Read the model definition and answer for the solid it produces. Units are mm, in the model's axes. A direction names the side the tool comes from. Coordinates: 2 decimals unless noted, no trailing zeros. Order: outer loops, then holes, each group sorted by start corner. A loop starts at its lowest first (then second) coordinate and runs counter-clockwise, first axis right, second up. Notation, with made-up numbers: M 68,1.25 L 97,1.25 A15 cw 97,10.25 Z; hole C 85,44.5 d10. An arc over 180 degrees is marked long. Write each question's results on one line, items separated by ' | '.
```python
from build123d import *

# Parameters (mm, degrees)
SKETCH_1_W             = 280
SKETCH_1_H             = 290
EXTRUDE_1_DEPTH        = 3
SKETCH_2_W             = 42
SKETCH_2_H             = 42
CUT_EXTRUDE_1_DEPTH    = 3
SKETCH_3_W             = 122
SKETCH_3_H             = 10
EXTRUDE_4_DEPTH        = 20
SKETCH_5_W             = 5
SKETCH_5_H             = 40
EXTRUDE_7_DEPTH        = 20
EXTRUDE_8_DEPTH        = 10
PATTERN_LINEAR_1_COUNT = 4
PATTERN_LINEAR_1_PITCH = 37.3
SKETCH_7_W             = 100
SKETCH_7_H             = 20
CUT_EXTRUDE_3_DEPTH    = 3
PATTERN_LINEAR_2_COUNT = 9
PATTERN_LINEAR_2_PITCH = 30
SKETCH_8_W             = 19.372377966
SKETCH_8_H             = 34.870206367
SKETCH_8_W_2           = 28.060398732
SKETCH_8_W_3           = 26.290591332
SKETCH_8_W_4           = 22.27663197
SKETCH_8_H_2           = 37.129793633
CUT_EXTRUDE_4_DEPTH    = 3


with BuildPart() as part:
    # 草图1 → 凸台-拉伸1 (new body)
    with BuildSketch(Plane(origin=(0, 0, 0), x_dir=(0, 0, -1), z_dir=(1, 0, 0))):
        with Locations((101.929406601, -104.613945148)):
            Rectangle(SKETCH_1_W, SKETCH_1_H)
    extrude(amount=EXTRUDE_1_DEPTH)

    # 草图2 → 切除-拉伸1 (cut)
    with BuildSketch(Plane.ZY):
        with Locations((-154.017718623, -48.907355815)):
            Rectangle(SKETCH_2_W, SKETCH_2_H)
    extrude(amount=-CUT_EXTRUDE_1_DEPTH, mode=Mode.SUBTRACT)

    # 草图3 → 凸台-拉伸4 (add)
    with BuildSketch(Plane.ZY):
        with Locations((-155.503619283, -115.067977161)):
            Rectangle(SKETCH_3_W, SKETCH_3_H)
    extrude(amount=EXTRUDE_4_DEPTH)

    # 草图5 → 凸台-拉伸7 (add)
    with BuildSketch(Plane.ZY):
        with Locations((-219.003619283, -10.067977161)):
            Rectangle(SKETCH_5_W, SKETCH_5_H)
        with Locations((-92.003619283, -10.067977161)):
            Rectangle(SKETCH_5_W, SKETCH_5_H)
    extrude(amount=EXTRUDE_7_DEPTH)

    # 草图6 → 凸台-拉伸8 (add)
    with BuildSketch(Plane.XY.offset(-94.503619283)):
        Polygon((-20, -120.067977161), (0, -120.067977161), (0, -140.067977161), align=None)
    extrude_8 = extrude(amount=-EXTRUDE_8_DEPTH)

    # 阵列(线性)1: 凸台-拉伸8 ×4
    with Locations(*[(0, 0, -i * PATTERN_LINEAR_1_PITCH) for i in range(1, PATTERN_LINEAR_1_COUNT)]):
        add(extrude_8)

    # 草图7 → 切除-拉伸3 (cut)
    with BuildSketch(Plane.ZY):
        with Locations((-22.758250254, 20.386054852)):
            Rectangle(SKETCH_7_W, SKETCH_7_H)
    cut_extrude_3 = extrude(amount=-CUT_EXTRUDE_3_DEPTH, mode=Mode.SUBTRACT)

    # 阵列(线性)2: 切除-拉伸3 ×9
    with Locations(*[(0, -i * PATTERN_LINEAR_2_PITCH, 0) for i in range(1, PATTERN_LINEAR_2_COUNT)]):
        add(cut_extrude_3, mode=Mode.SUBTRACT)

    # 草图8 → 切除-拉伸4 (cut)
    with BuildSketch(Plane.ZY):
        with Locations((-206.7174303, -172.090616985)):
            Rectangle(SKETCH_8_W, SKETCH_8_H)
        with Locations((-175.001041951, -172.090616985)):
            Rectangle(SKETCH_8_W_2, SKETCH_8_H)
        with Locations((-139.825546919, -172.090616985)):
            Rectangle(SKETCH_8_W_3, SKETCH_8_H)
        with Locations((-107.541935268, -172.090616985)):
            Rectangle(SKETCH_8_W_4, SKETCH_8_H)
        with Locations((-107.541935268, -216.090616985)):
            Rectangle(SKETCH_8_W_4, SKETCH_8_H_2)
        with Locations((-139.825546919, -216.090616985)):
            Rectangle(SKETCH_8_W_3, SKETCH_8_H_2)
        with Locations((-175.001041951, -216.090616985)):
            Rectangle(SKETCH_8_W_2, SKETCH_8_H_2)
        with Locations((-206.7174303, -216.090616985)):
            Rectangle(SKETCH_8_W, SKETCH_8_H_2)
    extrude(amount=-CUT_EXTRUDE_4_DEPTH, mode=Mode.SUBTRACT)


solid = part.part
```
(1) The part is cut by section C-C, the plane z = -8. Count the separate pieces of the cut face and the enclosed holes in it, then the cut area to 3 significant figures.
Conclusion:
separate pieces: 10 | enclosed holes: 0 | area: 330 mm²
(2) Given pin 1 (2.5 mm diameter, centred on x = -7.5, z = -220, fed in from +Y); pin 2 (1 mm diameter, centred on y = -38.5, z = -202, fed in from -X); pin 3 (12 mm diameter, centred on x = -12, y = 4, fed in from -Z); pin 4 (12 mm diameter, centred on x = -6.5, y = -87, fed in from -Z), each flat-ended and moving along its own axis, determine where each tip first touches the part or whether it passes through.
Conclusion:
pin 1: y = 9.93 | pin 2: x = 0 | pin 3: z = -221.5 | pin 4: through
(3) For faces 1 (the flat face through (-8, -128, -216.404)), 2 (the flat face through (-8, -122, -94.504)), 3 (the flat face through (-10, -120.068, -156)), determine the directions among +Z, -Z, +X, -X, +Y, -Y from which every point of the face is accessible in a straight line to the end or side of a thin tool.
Conclusion:
face 1: -Z, -X, -Y | face 2: +Z, -X, -Y | face 3: -X, -Y
(4) The part is cut by section B-B, the plane x = -6.5. Write down the section's boundary in (y, z), then the cut area to 3 significant figures.
Conclusion:
outline: M -133.57,-216.4 L -120.07,-216.4 L -120.07,-216.5 L -110.07,-216.5 L -110.07,-94.5 L -133.57,-94.5 L -133.57,-104.5 L -120.07,-104.5 L -120.07,-131.8 L -133.57,-131.8 L -133.57,-141.8 L -120.07,-141.8 L -120.07,-169.1 L -133.57,-169.1 L -133.57,-179.1 L -120.07,-179.1 L -120.07,-206.4 L -133.57,-206.4 Z; M -30.07,-221.5 L 9.93,-221.5 L 9.93,-216.5 L -30.07,-216.5 Z; M -30.07,-94.5 L 9.93,-94.5 L 9.93,-89.5 L -30.07,-89.5 Z | area: 2,160 mm²
(5) The part is cut by section A-A, the plane y = -100.5. Write down the section's boundary in (x, z).
Conclusion:
outline: M 0,-241.93 L 3,-241.93 L 3,-72.76 L 0,-72.76 Z; M 0,27.24 L 3,27.24 L 3,38.07 L 0,38.07 Z
(6) The part is cut by section D-D, the plane z = -82. Write down the section's boundary in (x, y), then the cut area to 3 significant figures.
Conclusion:
outline: M 0,-249.61 L 3,-249.61 L 3,40.39 L 0,40.39 Z | area: 870 mm²
(7) Straight lines are drawn through the part: line 1 (Z direction, x = 0.5, y = -223.5); line 2 (Z direction, x = -8, y = -125.5); line 3 (Z direction, x = 1.25, y = -43.5). For each, find the intervals that lie inside material, in ascending order.
Conclusion:
line 1: -241.93 to -216.4, -197.03 to -189.03, -160.97 to -152.97, -126.68 to -118.68, -96.4 to -72.76, 27.24 to 38.07 | line 2: -216.4 to -206.4, -179.1 to -169.1, -141.8 to -131.8, -104.5 to -94.5 | line 3: -241.93 to -175.02, -133.02 to -72.76, 27.24 to 38.07
